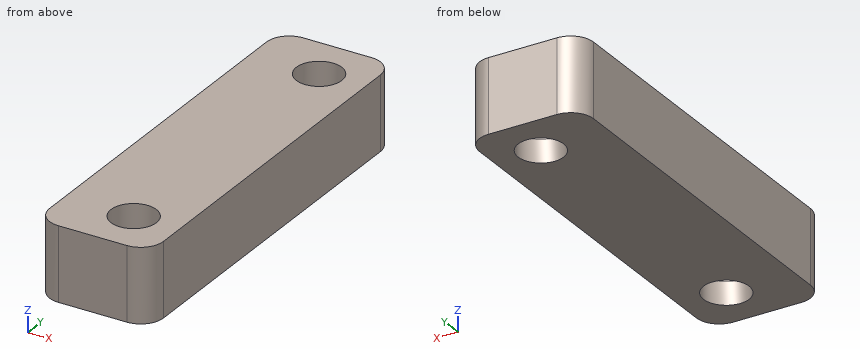
```python
from build123d import *

# Parameters (mm, degrees)
ESBO_O2_R                = 2
RESSALTO_EXTRUS_O1_DEPTH = 4.5
RESSALTO_EXTRUS_O2_START = 2
RESSALTO_EXTRUS_O2_DEPTH = 2
ESBO_O4_R                = 2
CORTE_EXTRUS_O2_DEPTH    = 37.976343789


with BuildPart() as part:
    # Esboço2 → Ressalto-extrusão1 (new body)
    with BuildSketch(Plane.XY):
        with BuildLine():
            Line((0, 2), (0, 33))
            ThreePointArc((0, 33), (0.585786438, 34.414213562), (2, 35))
            Line((2, 35), (8, 35))
            ThreePointArc((8, 35), (9.414213562, 34.414213562), (10, 33))
            Line((10, 33), (10, 2))
            ThreePointArc((10, 2), (9.414213562, 0.585786438), (8, 0))
            Line((8, 0), (2, 0))
            ThreePointArc((2, 0), (0.585786438, 0.585786438), (0, 2))
        make_face()
        with Locations((6, 4.25)):
            Circle(ESBO_O2_R, mode=Mode.SUBTRACT)
        with Locations((6, 30.75)):
            Circle(ESBO_O2_R, mode=Mode.SUBTRACT)
    extrude(amount=RESSALTO_EXTRUS_O1_DEPTH)

    # Esboço3 → Ressalto-extrusão2 (add)
    with BuildSketch(Plane(origin=(0, 0, 0), x_dir=(-1, 0, 0), z_dir=(0, 0, -1)).offset(RESSALTO_EXTRUS_O2_START)):
        with BuildLine():
            Line((0, 2), (0, 33))
            ThreePointArc((0, 33), (-0.585786438, 34.414213562), (-2, 35))
            Line((-2, 35), (-8, 35))
            ThreePointArc((-8, 35), (-9.414213562, 34.414213562), (-10, 33))
            Line((-10, 33), (-10, 2))
            ThreePointArc((-10, 2), (-9.414213562, 0.585786438), (-8, 0))
            Line((-8, 0), (-2, 0))
            ThreePointArc((-2, 0), (-0.585786438, 0.585786438), (0, 2))
        make_face()
    extrude(amount=-RESSALTO_EXTRUS_O2_DEPTH)

    # Esboço4 → Corte-extrusão2 (cut, through all)
    with BuildSketch(Plane.XY.offset(4.5)):
        with Locations((6, 4.25)):
            Circle(ESBO_O4_R)
        with Locations((6, 30.75)):
            Circle(ESBO_O4_R)
    extrude(amount=-CORTE_EXTRUS_O2_DEPTH, mode=Mode.SUBTRACT)


solid = part.part
```
Verification items for the finished model (mm, model axes). Round coordinates to 2 decimals unless told otherwise and drop trailing zeros. Write each loop counter-clockwise with the first axis right and the second up, starting at its lowest first coordinate (ties: lowest second). Pieces come first, ordered by that corner, then holes.
1. Gauge pin test, flat end, axial feed: P1, Ø3.5, axis at x = 6, y = 30.75, coming from the -Z side. Record the tip position at first contact, or that the pin passes through.
2. Section check D-D on y = 5. Enter the section's corners in (x, z).
3. Section check C-C on x = 6. Enter the section's corners in (y, z).
4. Scan lines: L1, parallel to Y at x = 6, z = -1.05; L2, parallel to Y at x = 7.5, z = 0.5; L3, parallel to X at y = 30, z = 3. Record each from-to range of solid material in increasing order.
5. Section check A-A on y = 30.75. Enter the section's corners in (x, z).
6. Section check B-B on z = 1.5. Enter the section's corners in (x, y).
Answer:
1. P1: passes through
2. outline: (0, -2) - (4.15, -2) - (4.15, 4.5) - (0, 4.5) - close; (7.85, -2) - (10, -2) - (10, 4.5) - (7.85, 4.5) - close
3. outline: (0, -2) - (2.25, -2) - (2.25, 4.5) - (0, 4.5) - close; (6.25, -2) - (28.75, -2) - (28.75, 4.5) - (6.25, 4.5) - close; (32.75, -2) - (35, -2) - (35, 4.5) - (32.75, 4.5) - close
4. L1: y = 0 to 2.25, 6.25 to 28.75, 32.75 to 35
4. L2: y = 0 to 2.93, 5.57 to 29.43, 32.07 to 35
4. L3: x = 0 to 4.15, 7.85 to 10
5. outline: (0, -2) - (4, -2) - (4, 4.5) - (0, 4.5) - close; (8, -2) - (10, -2) - (10, 4.5) - (8, 4.5) - close
6. outline: (0, 2) arc R2 ccw to (2, 0) - (8, 0) arc R2 ccw to (10, 2) - (10, 33) arc R2 ccw to (8, 35) - (2, 35) arc R2 ccw to (0, 33) - close; hole circle Ø4 at (6, 4.25); hole circle Ø4 at (6, 30.75)
